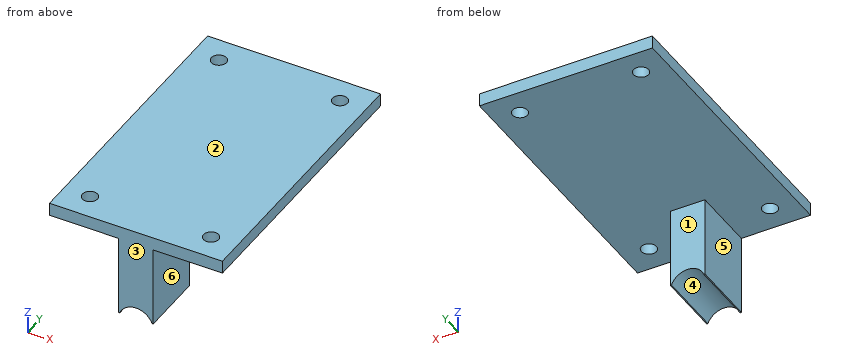
```python
from build123d import *

# Parameters (mm, degrees)
SKETCH1_W           = 40
SKETCH1_H           = 65
SKETCH1_R           = 1.75
BOSS_EXTRUDE1_DEPTH = 3
BOSS_EXTRUDE2_DEPTH = 15


with BuildPart() as part:
    # Sketch1 → Boss-Extrude1 (new body)
    with BuildSketch(Plane.XY):
        with Locations((20, 32.5)):
            Rectangle(SKETCH1_W, SKETCH1_H)
        with Locations((6, 59)):
            Circle(SKETCH1_R, mode=Mode.SUBTRACT)
        with Locations((34, 59)):
            Circle(SKETCH1_R, mode=Mode.SUBTRACT)
        with Locations((6, 6)):
            Circle(SKETCH1_R, mode=Mode.SUBTRACT)
        with Locations((34, 6)):
            Circle(SKETCH1_R, mode=Mode.SUBTRACT)
    extrude(amount=BOSS_EXTRUDE1_DEPTH)

    # Sketch2 → Boss-Extrude2 (add)
    with BuildSketch(Plane(origin=(0, 0, 0), x_dir=(-1, 0, 0), z_dir=(0, -1, 0))):
        with BuildLine():
            Line((-24, 0), (-16, 0))
            Line((-16, 0), (-16, 18.558164094))
            Line((-16, 18.558164094), (-16.268899731, 18.558164094))
            ThreePointArc((-16.268899731, 18.558164094), (-20, 16), (-23.731100269, 18.558164094))
            Line((-23.731100269, 18.558164094), (-24, 18.558164094))
            Line((-24, 18.558164094), (-24, 0))
        make_face()
    extrude(amount=-BOSS_EXTRUDE2_DEPTH)


solid = part.part
```
Can you work these out from the model? Positions are in its coordinate system, mm. Face numbers are marked on the shaded views. A direction names the side the tool comes from. Round coordinates to 2 decimals unless told otherwise and drop trailing zeros. Loops run counter-clockwise (first coordinate to the right, second up) from the corner with the lowest first, then second, coordinate; pieces in that order, holes last. Notation, with made-up numbers: M 49.5,22 L 65.5,22 A33 ccw 65.5,51 Z; hole C -17,38 d4. An arc over 180 degrees is marked long. Write item = value, one per line. Start each with the question number.
(1) Suppose I cut it at D-D on z = -6.5. Write out the boundary of the cut face in (x, y).
(2) Suppose I cut it at C-C on y = 6. Write out the boundary of the cut face in (x, z).
(3) Suppose I cut it at B-B on x = 6. Write out the boundary of the cut face in (y, z), plus the area to 3 significant figures.
(4) I'm going to push flat-ended pins straight in: P1, Ø12, axis at x = 11, y = 51.5, coming from the -Z side; P2, Ø3, axis at x = 34, y = 6, coming from the +Z side; P3, Ø12, axis at y = 11, z = -13, coming from the +X side; P4, Ø2.5, axis at x = 18.5, z = -10, coming from the +Y side. Where does each tip first touch, or does it pass through?
(5) Which directions (+Z, -Z, +X, -X, +Y, -Y) give clear straight access to the entire face, cutting with the end or side of a thin tool? Please do the marked faces 1 and 2.
(6) If we mould it in two halves opening along X, with no side actions, what happens to the marked faces 3, 4, 5 and 6? For each: released by +X, released by -X, zero draft, split by the parting line, or undercut.
(7) Suppose I cut it at A-A on y = 59. Write out the boundary of the cut face in (x, z).
(8) I need wall thicknesses on line 1 along Y through (x, z) = (6, 1.1); line 2 along Y through (x, z) = (4.5, 1.75); line 3 along Z through (x, y) = (32, 48). Which ranges of each line are inside material? Lowest first, please.
Answer block:
q1.outline = M 16,0 L 24,0 L 24,15 L 16,15 Z
q2.outline = M 0,0 L 4.25,0 L 4.25,3 L 0,3 Z; M 7.75,0 L 16,0 L 16,-18.56 L 16.27,-18.56 A4 cw 23.73,-18.56 L 24,-18.56 L 24,0 L 32.25,0 L 32.25,3 L 7.75,3 Z; M 35.75,0 L 40,0 L 40,3 L 35.75,3 Z
q3.outline = M 0,0 L 4.25,0 L 4.25,3 L 0,3 Z; M 7.75,0 L 57.25,0 L 57.25,3 L 7.75,3 Z; M 60.75,0 L 65,0 L 65,3 L 60.75,3 Z
q3.area = 174 mm²
q4.P1 = 0
q4.P2 = through
q4.P3 = 24
q4.P4 = 15
q5.face_1 = -Z, +X, -X, +Y
q5.face_2 = +Z, +X, -X, +Y, -Y
q6.face_3 = zero draft
q6.face_4 = undercut
q6.face_5 = released by -X
q6.face_6 = released by +X
q7.outline = M 0,0 L 4.25,0 L 4.25,3 L 0,3 Z; M 7.75,0 L 32.25,0 L 32.25,3 L 7.75,3 Z; M 35.75,0 L 40,0 L 40,3 L 35.75,3 Z
q8.line_1 = 0 to 4.25, 7.75 to 57.25, 60.75 to 65
q8.line_2 = 0 to 5.1, 6.9 to 58.1, 59.9 to 65
q8.line_3 = 0 to 3
